Geometry check sheet. Reference: the model listing, model coordinates, mm. Give positions to 0.01 mm unless a question says otherwise; leave off trailing zeros. Write each loop counter-clockwise with the first axis right and the second up, starting at its lowest first coordinate (ties: lowest second). Pieces come first, ordered by that corner, then holes. Notation, with made-up numbers: (-15.75, 44) -> (35.25, 44) arc R28 ccw to (35.25, 63) -> close; hole circle Ø8 at (48, 55). An arc over 180 degrees is marked (long way). Use a Markdown table: item, result. Add a question column.
from build123d import *

# Parameters (mm, degrees)
SKETCH1_W           = 170
SKETCH1_H           = 115
SKETCH1_W_2         = 166
SKETCH1_H_2         = 111
BOSS_EXTRUDE1_DEPTH = 2.75
SKETCH2_W           = 168
SKETCH2_H           = 113
CUT_EXTRUDE1_DEPTH  = 1.75
CHAMFER1_SIZE       = 0.5


with BuildPart() as part:
    # Sketch1 → Boss-Extrude1 (new body)
    with BuildSketch(Plane(origin=(0, 0, 0), x_dir=(1, 0, 0), z_dir=(0, 1, 0))):
        with Locations((85, 57.5)):
            Rectangle(SKETCH1_W, SKETCH1_H)
        with Locations((85, 57.5)):
            Rectangle(SKETCH1_W_2, SKETCH1_H_2, mode=Mode.SUBTRACT)
    extrude(amount=BOSS_EXTRUDE1_DEPTH)

    # Sketch2 → Cut-Extrude1 (cut)
    with BuildSketch(Plane(origin=(0, 2.75, 0), x_dir=(1, 0, 0), z_dir=(0, 1, 0))):
        with Locations((85, 57.5)):
            Rectangle(SKETCH2_W, SKETCH2_H)
    extrude(amount=-CUT_EXTRUDE1_DEPTH, mode=Mode.SUBTRACT)

    # Chamfer1
    chamfer1_edges = [part.edges().sort_by_distance(p)[0] for p in [
        (2, 0, -57.5),
        (85, 0, -2),
        (168, 0, -57.5),
        (85, 0, -113),
        (85, 0, -115),
        (170, 0, -57.5),
        (85, 0, 0),
        (0, 0, -57.5),
    ]]
    chamfer(chamfer1_edges, length=CHAMFER1_SIZE)


solid = part.part
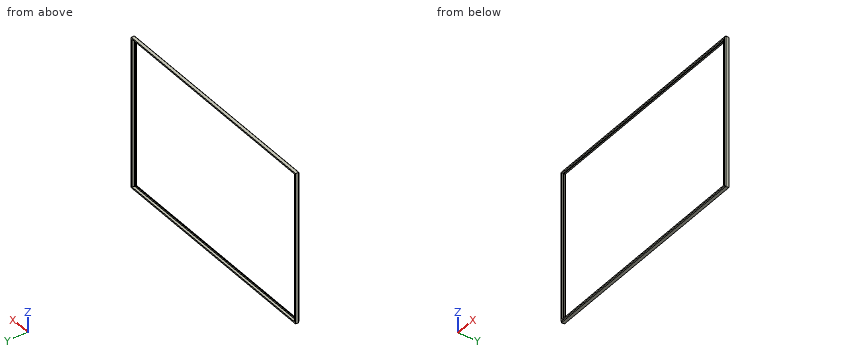
1) Material ranges on probe 1 along Z at (x, y) = (15, 2.3); probe 2 along X at (y, z) = (0.7, -47); probe 3 along Z at (x, y) = (23, 0.9), recorded low to high. Write a range as [from, to].
2) Sectioned sample at C-C, the plane z = -61. Enter the section's corners in (x, y).
3) Sectioned sample at B-B, the plane x = 154. Enter the section's corners in (y, z), and give its area (3 significant figures).
4) Sectioned sample at A-A, the plane y = 1.7. Enter the section's corners in (x, z), and give its area (3 significant figures).
Check values:
| question | item | result |
|---|---|---|
| 1 | probe 1 | [-115, -114], [-1, 0] |
| 1 | probe 2 | [0, 2], [168, 170] |
| 1 | probe 3 | [-115, -113], [-2, 0] |
| 2 | outline | (0, 0.5) -> (0.5, 0) -> (1.5, 0) -> (2, 0.5) -> (2, 1) -> (1, 1) -> (1, 2.75) -> (0, 2.75) -> close; (168, 0.5) -> (168.5, 0) -> (169.5, 0) -> (170, 0.5) -> (170, 2.75) -> (169, 2.75) -> (169, 1) -> (168, 1) -> close |
| 3 | outline | (0, -114.5) -> (0.5, -115) -> (2.75, -115) -> (2.75, -114) -> (1, -114) -> (1, -113) -> (0.5, -113) -> (0, -113.5) -> close; (0, -1.5) -> (0.5, -2) -> (1, -2) -> (1, -1) -> (2.75, -1) -> (2.75, 0) -> (0.5, 0) -> (0, -0.5) -> close |
| 3 | area | 7.00 mm² |
| 4 | outline | (0, -115) -> (170, -115) -> (170, 0) -> (0, 0) -> close; hole (1, -114) -> (169, -114) -> (169, -1) -> (1, -1) -> close |
| 4 | area | 566 mm² |
